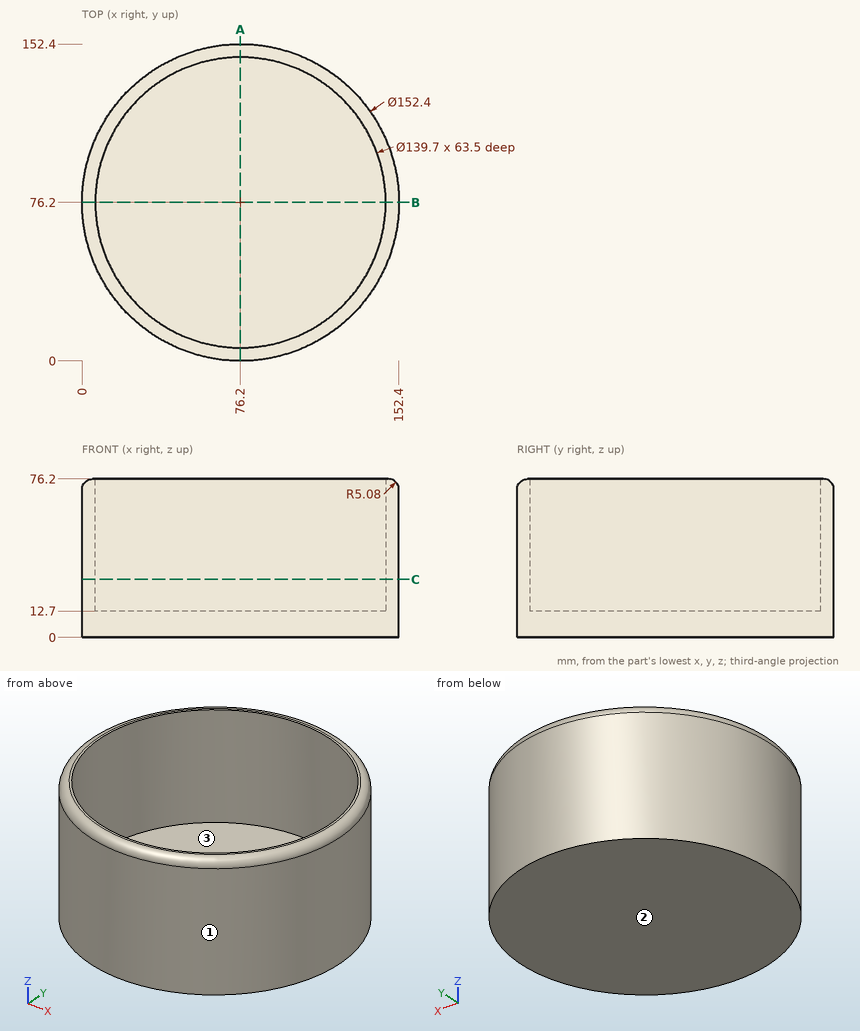
Drawing for the job (mm, zero at the part's lowest x, y, z). Round coordinates to 2 decimals unless told otherwise and drop trailing zeros. Write each loop counter-clockwise with the first axis right and the second up, starting at its lowest first coordinate (ties: lowest second). Pieces come first, ordered by that corner, then holes. Notation, with made-up numbers: M 53.5,-4 L 104.5,-4 A33 cw 104.5,24 Z; hole C 79,10.25 d11. An arc over 180 degrees is marked long. Answer as a JSON object with one key per item and string values. Group by question number.
(1) Flat gauge pins, fed straight in: pin 1 (8 mm diameter, centred on x = 79, z = 31, fed in from -Y); pin 2 (3 mm diameter, centred on x = 33.5, z = 43, fed in from +Y); pin 3 (8 mm diameter, centred on y = 105, z = 36.5, fed in from -X). Where does each tip first touch, or does it go through?
(2) Mould opens along Z. For the marked faces 1, 2 and 3 say: pulls with the +Z half, pulls with the -Z half, needs draft (parallel to the pull), parting line crosses it, or undercut.
(3) Cut at A-A (x = 76.2). Give the cut face in (y, z), and give its area (3 significant figures).
(4) Cut at C-C (z = 28). Give the cut face in (x, y).
(5) Drill centre lines: L1, parallel to X at y = 76, z = 48; L2, parallel to Z at x = 115, y = 98. Where is each one in solid material? Low to high.
Responses:
{
 "1": {"pin 1": "stops at y = 0", "pin 2": "stops at y = 140.3", "pin 3": "stops at x = 4.15"},
 "2": {"face 1": "needs draft", "face 2": "pulls with the -Z half", "face 3": "pulls with the +Z half"},
 "3": {"outline": "M 0,0 L 152.4,0 L 152.4,71.12 A5.08 ccw 147.32,76.2 L 146.05,76.2 L 146.05,12.7 L 6.35,12.7 L 6.35,76.2 L 5.08,76.2 A5.08 ccw 0,71.12 Z", "area": "2,730 mm2"},
 "4": {"outline": "C 76.2,76.2 d152.4; hole C 76.2,76.2 d139.7"},
 "5": {"L1": "x = 0 to 6.35, 146.05 to 152.4", "L2": "z = 0 to 12.7"}
}
